Work out the finished part from the listing and answer in its coordinate system (mm). A direction names the side the tool comes from. Coordinates: 2 decimals unless noted, no trailing zeros. Write each loop counter-clockwise with the first axis right and the second up, starting at its lowest first coordinate (ties: lowest second). Pieces come first, ordered by that corner, then holes. Notation, with made-up numbers: (18, 64) - (23, 64) arc R27 cw to (23, 97) - close; hole circle Ø10 at (74, 83.25). An arc over 180 degrees is marked (long way). One line per item, written item: value.
```python
from build123d import *

# Parameters (mm, degrees)
SKETCH2_W              = 293.6875
SKETCH2_H              = 52.578
BOSS_EXTRUDE1_DEPTH    = 5.334
SKETCH3_W              = 25.4
SKETCH3_H              = 5.334
BOSS_EXTRUDE2_DEPTH    = 5.334
SKETCH4_R              = 1.27
BBQ_SKEWER_HOLES_DEPTH = 53.578


with BuildPart() as part:
    # Sketch2 → Boss-Extrude1 (new body)
    with BuildSketch(Plane(origin=(0, 0, 0), x_dir=(1, 0, 0), z_dir=(0, 1, 0))):
        Rectangle(SKETCH2_W, SKETCH2_H)
    extrude(amount=BOSS_EXTRUDE1_DEPTH)

    # Sketch3 → Boss-Extrude2 (add)
    with BuildSketch(Plane.XY.offset(26.289)):
        Polygon((184.94375, 36.1188), (146.84375, 5.334), (-146.84375, 5.334), (-146.84375, 36.1188), (146.84375, 36.1188), align=None)
        with Locations((-32.54375, 38.7858)):
            Rectangle(SKETCH3_W, SKETCH3_H)
        Polygon((146.84375, 36.1188), (159.54375, 36.1188), (159.54375, 41.4528), (134.14375, 41.4528), (134.14375, 36.1188), align=None)
    boss_extrude2 = extrude(amount=-BOSS_EXTRUDE2_DEPTH)

    # Mirror1: Boss-Extrude2 across plane
    add(boss_extrude2.mirror(Plane.XY))

    # Sketch4 → BBQ Skewer Holes (cut, through all)
    with BuildSketch(Plane.XY.offset(26.289)):
        with Locations((110.744734301, 22.342412484)):
            Circle(SKETCH4_R)
    extrude(amount=-BBQ_SKEWER_HOLES_DEPTH, mode=Mode.SUBTRACT)


solid = part.part
```
Item 1: Determine the mould class of faces 1 (the face through (-45.244, 39, -24)), 2 (the face through (-2, 0, 0)), 3 (the face through (134.144, 39, -24)) for opening direction X: +X half, -X half, draft (parallel to the pull), parting line (faces both ways), or undercut.
Evaluation:
face 1: -X half
face 2: draft
face 3: undercut
Item 2: Consider probe 1 along Z at (x, y) = (-6.5, 32) (3 decimals); probe 2 along Y at (x, z) = (60.5, -8); probe 3 along X at (y, z) = (2.5, 0). Determine where each line is inside the solid, lowest interval first.
Evaluation:
probe 1: z = -26.289 to -20.955, 20.955 to 26.289
probe 2: y = 0 to 5.33
probe 3: x = -146.84 to 146.84
Item 3: Given pin 1 (2.5 mm diameter, centred on x = 68.5, z = -23.5, fed in from +Y); pin 2 (6 mm diameter, centred on y = 4.5, z = 17.5, fed in from +X); pin 3 (1.5 mm diameter, centred on x = -47.5, z = -1.5, fed in from +Y), each flat-ended and moving along its own axis, determine where each tip first touches the part or whether it passes through.
Evaluation:
pin 1: stops at y = 36.12
pin 2: stops at x = 146.84
pin 3: stops at y = 5.33
Item 4: Section A-A, the plane x = 117 is taken. Determine the outline of the cut face in (y, z) (3 decimals).
Evaluation:
outline: (0, -26.289) - (36.119, -26.289) - (36.119, -20.955) - (5.334, -20.955) - (5.334, 20.955) - (36.119, 20.955) - (36.119, 26.289) - (0, 26.289) - close
Item 5: Section C-C, the plane z = 0 is taken. Determine the outline of the cut face in (x, y).
Evaluation:
outline: (-146.84, 0) - (146.84, 0) - (146.84, 5.33) - (-146.84, 5.33) - close
Item 6: Which of the six approach directions +Z, -Z, +X, -X, +Y, -Y give full straight-line access (tool end or side, diameter ignored) to faces 4 (the face through (21, 24, 20.955)), 5 (the face through (172, 36.119, -24)), 6 (the face through (-19.844, 39, -24))?
Evaluation:
face 4: +X, -X, +Y
face 5: +Z, -Z, +X, +Y
face 6: +Z, -Z, +Y
Item 7: Section B-B, the plane y = 18 is taken. Determine the outline of the cut face in (x, z) (1 decimal), then the cut area to 3 significant figures.
Evaluation:
outline: (-146.8, -26.3) - (162.5, -26.3) - (162.5, -21) - (-146.8, -21) - close; (-146.8, 21) - (162.5, 21) - (162.5, 26.3) - (-146.8, 26.3) - close
area: 3,300 mm2
